```python
from build123d import *

# Parameters (mm, degrees)
F0_R      = 2.345
F1_DEPTH  = 11.94
F2_DEPTH  = 11.94
F5_DEPTH  = 166.5
F6_DEPTH  = 12.5
F7_W      = 0.5
F7_H      = 1.86
F4_W      = 1
F4_H      = 6.89
F9_DEPTH  = 12.5
F10_R     = 2
F11_DEPTH = 20.5
F12_W     = 0.2
F12_H     = 0.4
F14_DEPTH = 12.5
F15_DEPTH = 25
F16_DEPTH = 12.5
F17_R     = 0.4999


# Not quite as in the source:
# - a fillet or chamfer is up to 0.001 mm smaller than in the source, because OpenCascade refuses the exact size
# - a pattern or mirror of a feature is missing from the dataset's text; its kind, count and spacing are read off the source's solid


with BuildPart() as f1:
    # F0 (on Top) → F1 (new body)
    with BuildSketch(Plane.XY):
        Circle(F0_R)
    extrude(amount=F1_DEPTH)

    # F0 (on Top) → F2 (join)
    with BuildSketch(Plane.XY):
        Circle(F0_R)
    extrude(amount=-F2_DEPTH)

    # F3 (on Front) → F5 (cut, symmetric)
    with BuildSketch(Plane.XZ):
        with BuildLine():
            Line((-0.545, -12.9641438561), (0.545, -12.9641438561))
            Line((0.545, -12.9641438561), (0.545, -9.629))
            ThreePointArc((0.545, -9.629), (0, -10.174), (-0.545, -9.629))
            Line((-0.545, -9.629), (-0.545, -12.9641438561))
        make_face()
        with BuildLine():
            ThreePointArc((-0.545, -9.629), (0, -10.174), (0.545, -9.629))
            Line((0.545, -9.629), (-0.545, -9.629))
        make_face()
        with BuildLine():
            Line((-0.545, -9.629), (0.545, -9.629))
            ThreePointArc((0.545, -9.629), (0, -9.084), (-0.545, -9.629))
        make_face()
        with BuildLine():
            ThreePointArc((-0.545, 9.629), (0, 9.084), (0.545, 9.629))
            ThreePointArc((0.545, 9.629), (0, 10.174), (-0.545, 9.629))
        make_face()
        with BuildLine():
            ThreePointArc((-0.545, 9.629), (0, 10.174), (0.545, 9.629))
            Line((0.545, 9.629), (0.545, 12.9641438561))
            Line((0.545, 12.9641438561), (-0.545, 12.9641438561))
            Line((-0.545, 12.9641438561), (-0.545, 9.629))
        make_face()
    extrude(amount=F5_DEPTH, both=True, mode=Mode.SUBTRACT)

    # F3 (on Front) → F6 (cut, symmetric)
    with BuildSketch(Plane.XZ):
        with BuildLine():
            Line((-0.545, -12.9641438561), (0.545, -12.9641438561))
            Line((0.545, -12.9641438561), (0.545, -9.629))
            ThreePointArc((0.545, -9.629), (0, -10.174), (-0.545, -9.629))
            Line((-0.545, -9.629), (-0.545, -12.9641438561))
        make_face()
        with BuildLine():
            ThreePointArc((-0.545, -9.629), (0, -10.174), (0.545, -9.629))
            Line((0.545, -9.629), (-0.545, -9.629))
        make_face()
        with BuildLine():
            Line((-0.545, -9.629), (0.545, -9.629))
            ThreePointArc((0.545, -9.629), (0, -9.084), (-0.545, -9.629))
        make_face()
        with BuildLine():
            ThreePointArc((-0.545, 9.629), (0, 9.084), (0.545, 9.629))
            ThreePointArc((0.545, 9.629), (0, 10.174), (-0.545, 9.629))
        make_face()
        with BuildLine():
            ThreePointArc((-0.545, 9.629), (0, 10.174), (0.545, 9.629))
            Line((0.545, 9.629), (0.545, 12.9641438561))
            Line((0.545, 12.9641438561), (-0.545, 12.9641438561))
            Line((-0.545, 12.9641438561), (-0.545, 9.629))
        make_face()
    extrude(amount=F6_DEPTH, both=True, mode=Mode.SUBTRACT)

    # F7 (on Front) → F8 (revolve)
    with BuildSketch(Plane.XZ):
        with Locations((-2.5410750752, -4.01)):
            Rectangle(F7_W, F7_H)
    revolve(axis=Axis((0, 0, 0), (0, 0, -1)))

    # F4 (on Right) → F9 (cut, symmetric)
    with BuildSketch(Plane.YZ):
        with Locations((0, -4.195)):
            Rectangle(F4_W, F4_H)
        with Locations((0, 4.195)):
            Rectangle(F4_W, F4_H)
    extrude(amount=F9_DEPTH, both=True, mode=Mode.SUBTRACT)

    # F10 (on Top) → F11 (cut, symmetric)
    with BuildSketch(Plane.XY):
        Circle(F10_R)
    extrude(amount=F11_DEPTH, both=True, mode=Mode.SUBTRACT)

    # F12 (on Right) → F13 (revolve)
    with BuildSketch(Plane.YZ):
        with Locations((2.380789337, 11.74)):
            Rectangle(F12_W, F12_H)
    f13 = revolve(axis=Axis((0, 0, 0), (0, 0, -1)))

    # F13_copies: F13 across plane
    add(f13.mirror(Plane(origin=(0, 0, 0), x_dir=(-1, 0, 0), z_dir=(0, 0, -1))))

    # F3 (on Front) → F14 (cut, symmetric)
    with BuildSketch(Plane.XZ):
        with BuildLine():
            Line((-0.545, -12.9641438561), (0.545, -12.9641438561))
            Line((0.545, -12.9641438561), (0.545, -9.629))
            ThreePointArc((0.545, -9.629), (0, -10.174), (-0.545, -9.629))
            Line((-0.545, -9.629), (-0.545, -12.9641438561))
        make_face()
        with BuildLine():
            ThreePointArc((-0.545, -9.629), (0, -10.174), (0.545, -9.629))
            Line((0.545, -9.629), (-0.545, -9.629))
        make_face()
        with BuildLine():
            Line((-0.545, -9.629), (0.545, -9.629))
            ThreePointArc((0.545, -9.629), (0, -9.084), (-0.545, -9.629))
        make_face()
        with BuildLine():
            ThreePointArc((-0.545, 9.629), (0, 9.084), (0.545, 9.629))
            ThreePointArc((0.545, 9.629), (0, 10.174), (-0.545, 9.629))
        make_face()
        with BuildLine():
            ThreePointArc((-0.545, 9.629), (0, 10.174), (0.545, 9.629))
            Line((0.545, 9.629), (0.545, 12.9641438561))
            Line((0.545, 12.9641438561), (-0.545, 12.9641438561))
            Line((-0.545, 12.9641438561), (-0.545, 9.629))
        make_face()
    extrude(amount=F14_DEPTH, both=True, mode=Mode.SUBTRACT)

    # F3 (on Front) → F15 (cut)
    with BuildSketch(Plane.XZ):
        with BuildLine():
            Line((-0.545, -12.9641438561), (0.545, -12.9641438561))
            Line((0.545, -12.9641438561), (0.545, -9.629))
            ThreePointArc((0.545, -9.629), (0, -10.174), (-0.545, -9.629))
            Line((-0.545, -9.629), (-0.545, -12.9641438561))
        make_face()
        with BuildLine():
            ThreePointArc((-0.545, -9.629), (0, -10.174), (0.545, -9.629))
            Line((0.545, -9.629), (-0.545, -9.629))
        make_face()
        with BuildLine():
            Line((-0.545, -9.629), (0.545, -9.629))
            ThreePointArc((0.545, -9.629), (0, -9.084), (-0.545, -9.629))
        make_face()
        with BuildLine():
            ThreePointArc((-0.545, 9.629), (0, 9.084), (0.545, 9.629))
            ThreePointArc((0.545, 9.629), (0, 10.174), (-0.545, 9.629))
        make_face()
        with BuildLine():
            ThreePointArc((-0.545, 9.629), (0, 10.174), (0.545, 9.629))
            Line((0.545, 9.629), (0.545, 12.9641438561))
            Line((0.545, 12.9641438561), (-0.545, 12.9641438561))
            Line((-0.545, 12.9641438561), (-0.545, 9.629))
        make_face()
    extrude(amount=-F15_DEPTH, mode=Mode.SUBTRACT)

    # F3 (on Front) → F16 (cut, symmetric)
    with BuildSketch(Plane.XZ):
        with BuildLine():
            Line((-0.545, -12.9641438561), (0.545, -12.9641438561))
            Line((0.545, -12.9641438561), (0.545, -9.629))
            ThreePointArc((0.545, -9.629), (0, -10.174), (-0.545, -9.629))
            Line((-0.545, -9.629), (-0.545, -12.9641438561))
        make_face()
        with BuildLine():
            ThreePointArc((-0.545, -9.629), (0, -10.174), (0.545, -9.629))
            Line((0.545, -9.629), (-0.545, -9.629))
        make_face()
        with BuildLine():
            Line((-0.545, -9.629), (0.545, -9.629))
            ThreePointArc((0.545, -9.629), (0, -9.084), (-0.545, -9.629))
        make_face()
        with BuildLine():
            ThreePointArc((-0.545, 9.629), (0, 9.084), (0.545, 9.629))
            ThreePointArc((0.545, 9.629), (0, 10.174), (-0.545, 9.629))
        make_face()
        with BuildLine():
            ThreePointArc((-0.545, 9.629), (0, 10.174), (0.545, 9.629))
            Line((0.545, 9.629), (0.545, 12.9641438561))
            Line((0.545, 12.9641438561), (-0.545, 12.9641438561))
            Line((-0.545, 12.9641438561), (-0.545, 9.629))
        make_face()
    extrude(amount=F16_DEPTH, both=True, mode=Mode.SUBTRACT)

    # F17 (radius 0.5 in the source; OpenCascade refuses exactly that, so slightly less here)
    f17_edges = [f1.edges().sort_by_distance(p)[0] for p in [
        (2.113783, 0.5, 0.75),
        (-2.113783, 0.5, 0.75),
        (2.113783, -0.5, 0.75),
        (-2.113783, -0.5, 0.75),
        (2.113783, -0.5, -0.75),
        (-2.113783, -0.5, -0.75),
        (2.113783, 0.5, -0.75),
        (-2.113783, 0.5, -0.75),
        (-2.113783, -0.5, -7.64),
        (2.113783, -0.5, -7.64),
        (2.113783, 0.5, -7.64),
        (-2.113783, 0.5, -7.64),
        (2.113783, -0.5, 7.64),
        (-2.113783, -0.5, 7.64),
        (2.113783, 0.5, 7.64),
        (-2.113783, 0.5, 7.64),
    ]]
    fillet(f17_edges, radius=F17_R)


solid = f1.part
```
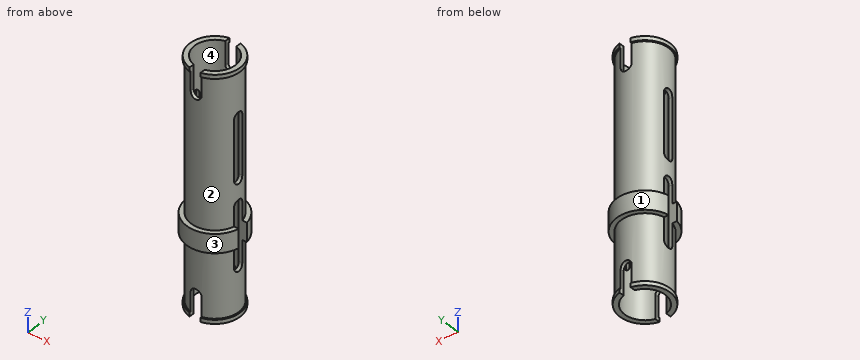
Part model, mm, in its own coordinate system. Face numbers are marked on the shaded views. Coordinates: 2 decimals unless noted, no trailing zeros. Order: outer loops, then holes, each group sorted by start corner. A loop starts at its lowest first (then second) coordinate and runs counter-clockwise, first axis right, second up. Notation, with made-up numbers: (88.5, -16.5) - (137.5, -16.5) arc R13 cw to (137.5, -1.5) - close; hole circle Ø5 at (-21.75, 31.25). An arc over 180 degrees is marked (long way). Return JSON: item names as keys, results as strings. Group by question number.
Item 1: Cut at B-B (x = 0). List the corners of the cut face in (y, z) (3 decimals).
Item 2: Cut at C-C (y = -1.2). List the corners of the cut face in (x, z), plus the area to 3 significant figures.
Item 3: Drill centre lines: probe 1 along Z at (x, y) = (-2.2, -0.95); probe 2 along X at (y, z) = (0, 0.25) (3 decimals). Where is each one in solid material? Low to high. Write a range as from..to.
Item 4: Pull direction Y, two halves, no side cores. Call the marked faces 1, 2, 3 and 4: pulls with the +Y half, pulls with the -Y half, needs draft (parallel to the pull), parting line crosses it, or undercut.
Item 5: Pin check, flat tips, straight feed: pin 1 (3 mm diameter, centred on x = -2, z = 4.5, fed in from +Y); pin 2 (0.5 mm diameter, centred on y = -2, z = -11.5, fed in from +X); pin 3 (0.5 mm diameter, centred on y = -2, z = 10.5, fed in from -X). Stop position of each tip, or through.
Item 6: Cut at D-D (z = -10.5). List the corners of the cut face in (x, y) (3 decimals).
Check values:
{
 "1": {"outline": "(-2.791, -4.94) - (-2.345, -4.94) - (-2.345, -9.084) - (-2, -9.084) - (-2, 9.084) - (-2.345, 9.084) - (-2.345, -3.08) - (-2.791, -3.08) - close; (2, -9.084) - (2.345, -9.084) - (2.345, -4.94) - (2.791, -4.94) - (2.791, -3.08) - (2.345, -3.08) - (2.345, 9.084) - (2, 9.084) - close"},
 "2": {"outline": "(-2.52, -4.94) - (-2.01, -4.94) - (-2.01, -11.54) - (-2.17, -11.54) - (-2.17, -11.94) - (-1.6, -11.94) - (-1.6, 11.94) - (-2.17, 11.94) - (-2.17, 11.54) - (-2.01, 11.54) - (-2.01, -3.08) - (-2.52, -3.08) - close; (1.6, -11.94) - (2.17, -11.94) - (2.17, -11.54) - (2.01, -11.54) - (2.01, -4.94) - (2.52, -4.94) - (2.52, -3.08) - (2.01, -3.08) - (2.01, 11.54) - (2.17, 11.54) - (2.17, 11.94) - (1.6, 11.94) - close", "area": "21.9 mm2"},
 "3": {"probe 1": "z = -11.94..-11.54, -4.94..-3.08, 11.54..11.94", "probe 2": "x = -2.345..-2, 2..2.345"},
 "4": {"face 1": "pulls with the +Y half", "face 2": "parting line crosses it", "face 3": "pulls with the -Y half", "face 4": "undercut"},
 "5": {"pin 1": "stops at y = 2.29", "pin 2": "stops at x = 1.76", "pin 3": "stops at x = -1.56"},
 "6": {"outline": "(-0.545, -2.281) - (-0.545, -1.924) arc R2 cw to (-0.545, 1.924) - (-0.545, 2.281) arc R2.345 ccw to start; (0.545, -2.281) arc R2.345 ccw to (0.545, 2.281) - (0.545, 1.924) arc R2 cw to (0.545, -1.924) - close"}
}
